For this review, take the finished solid that the model builds, in its own axes (mm). Face numbers are marked on the shaded views. Give positions to 0.01 mm unless a question says otherwise; leave off trailing zeros. Write each loop counter-clockwise with the first axis right and the second up, starting at its lowest first coordinate (ties: lowest second). Pieces come first, ordered by that corner, then holes. Notation, with made-up numbers: M -25,88 L 31,88 A17 cw 31,105 Z; hole C -14.5,-6.5 d5. An arc over 180 degrees is marked long. One line per item, written item: value. Start each with the question number.
Item 1: Consider section A-A, the plane x = 0. Write out the cut boundary in (y, z), and give its area (3 significant figures).
Item 2: Consider section B-B, the plane z = 6.5. Give the number of separate pieces and of enclosed holes in the cut face, and give its area (3 significant figures).
Item 3: Mouldability with a two-part tool opening along X and no side actions: class the marked faces 1 and 2 as released by +X, released by -X, zero draft, split by the parting line, or undercut.
Item 4: To check wall thickness, follow probe 1 along X at (y, z) = (1, 9.25); probe 2 along X at (y, z) = (-29, 6.75); probe 3 along Y at (x, z) = (-25, 4). State the ranges of each line that lie inside material, in increasing order.
Item 5: Clearance check with flat-ended pins moving along their axes: pin 1 Ø5 at (y, z) = (27.5, 5.5) entering from -X; pin 2 Ø5 at (x, y) = (25.5, -5) entering from +Z; pin 3 Ø4 at (y, z) = (-27, 7) entering from +X; pin 4 Ø3 at (x, z) = (-32, 1.5) entering from -Y. State where each tip first meets the part, or that it passes through.
```python
from build123d import *

# Parameters (mm, degrees)
SKETCH_8_R      = 5.308589755
SKETCH_8_R_2    = 9.5
EXTRUDE_1_DEPTH = 10


with BuildPart() as part:
    # 草图8 → 凸台-拉伸1 (new body)
    with BuildSketch(Plane.XY):
        with BuildLine():
            ThreePointArc((44.955555556, -1.999506112), (43, 0), (44.955555556, 1.999506112))
            ThreePointArc((44.955555556, 1.999506112), (44.861280018, 3.530659308), (44.714869736, 5.05770941))
            ThreePointArc((44.714869736, 5.05770941), (42.470598646, 6.726681997), (44.089286398, 9.007487158))
            ThreePointArc((44.089286398, 9.007487158), (43.756646418, 10.505041374), (43.373155424, 11.990387341))
            ThreePointArc((43.373155424, 11.990387341), (40.895430201, 13.287730758), (42.137392686, 15.793673975))
            ThreePointArc((42.137392686, 15.793673975), (41.574578963, 17.220754456), (40.963450077, 18.627822142))
            ThreePointArc((40.963450077, 18.627822142), (38.31328054, 19.521591489), (39.14793652, 22.190968124))
            ThreePointArc((39.14793652, 22.190968124), (38.368807396, 23.512435412), (37.54508864, 24.806578139))
            ThreePointArc((37.54508864, 24.806578139), (34.787730758, 25.274765849), (35.194528232, 28.041846989))
            ThreePointArc((35.194528232, 28.041846989), (34.218268452, 29.225162175), (33.202242516, 30.374513855))
            ThreePointArc((33.202242516, 30.374513855), (30.405591591, 30.405591591), (30.374513855, 33.202242516))
            ThreePointArc((30.374513855, 33.202242516), (29.225162175, 34.218268452), (28.041846989, 35.194528232))
            ThreePointArc((28.041846989, 35.194528232), (25.274765849, 34.787730758), (24.806578139, 37.54508864))
            ThreePointArc((24.806578139, 37.54508864), (23.512435412, 38.368807396), (22.190968124, 39.14793652))
            ThreePointArc((22.190968124, 39.14793652), (19.521591489, 38.31328054), (18.627822142, 40.963450077))
            ThreePointArc((18.627822142, 40.963450077), (17.220754456, 41.574578963), (15.793673975, 42.137392686))
            ThreePointArc((15.793673975, 42.137392686), (13.287730758, 40.895430201), (11.990387341, 43.373155424))
            ThreePointArc((11.990387341, 43.373155424), (10.505041374, 43.756646418), (9.007487158, 44.089286398))
            ThreePointArc((9.007487158, 44.089286398), (6.726681997, 42.470598646), (5.05770941, 44.714869736))
            ThreePointArc((5.05770941, 44.714869736), (3.530659308, 44.861280018), (1.999506112, 44.955555556))
            ThreePointArc((1.999506112, 44.955555556), (0, 43), (-1.999506112, 44.955555556))
            ThreePointArc((-1.999506112, 44.955555556), (-3.530659308, 44.861280018), (-5.05770941, 44.714869736))
            ThreePointArc((-5.05770941, 44.714869736), (-5.044095711, 44.580728744), (-5.039550927, 44.445975327))
            ThreePointArc((-5.039550927, 44.445975327), (-6.860487337, 42.454007398), (-9.007487158, 44.089286398))
            ThreePointArc((-9.007487158, 44.089286398), (-10.505041374, 43.756646418), (-11.990387341, 43.373155424))
            ThreePointArc((-11.990387341, 43.373155424), (-11.927033485, 43.088442863), (-11.905764747, 42.797543233))
            ThreePointArc((-11.905764747, 42.797543233), (-13.570965148, 40.825765044), (-15.793673975, 42.137392686))
            ThreePointArc((-15.793673975, 42.137392686), (-17.220754456, 41.574578963), (-18.627822142, 40.963450077))
            ThreePointArc((-18.627822142, 40.963450077), (-18.479764717, 40.540545937), (-18.429572488, 40.095293588))
            ThreePointArc((-18.429572488, 40.095293588), (-19.941101031, 38.155861807), (-22.190968124, 39.14793652))
            ThreePointArc((-22.190968124, 39.14793652), (-23.512435412, 38.368807396), (-24.806578139, 37.54508864))
            ThreePointArc((-24.806578139, 37.54508864), (-24.541473285, 37.002624685), (-24.450336353, 36.405764747))
            ThreePointArc((-24.450336353, 36.405764747), (-25.811204626, 34.510636615), (-28.041846989, 35.194528232))
            ThreePointArc((-28.041846989, 35.194528232), (-29.225162175, 34.218268452), (-30.374513855, 33.202242516))
            ThreePointArc((-30.374513855, 33.202242516), (-29.963655564, 32.564592842), (-29.819805153, 31.819805153))
            ThreePointArc((-29.819805153, 31.819805153), (-31.033953617, 29.980664767), (-33.202242516, 30.374513855))
            ThreePointArc((-33.202242516, 30.374513855), (-34.218268452, 29.225162175), (-35.194528232, 28.041846989))
            ThreePointArc((-35.194528232, 28.041846989), (-34.613772416, 27.338459928), (-34.405764747, 26.450336353))
            ThreePointArc((-34.405764747, 26.450336353), (-35.478038437, 24.678522623), (-37.54508864, 24.806578139))
            ThreePointArc((-37.54508864, 24.806578139), (-38.368807396, 23.512435412), (-39.14793652, 22.190968124))
            ThreePointArc((-39.14793652, 22.190968124), (-38.378506744, 21.455556373), (-38.095293588, 20.429572488))
            ThreePointArc((-38.095293588, 20.429572488), (-39.031412246, 18.736009236), (-40.963450077, 18.627822142))
            ThreePointArc((-40.963450077, 18.627822142), (-41.574578963, 17.220754456), (-42.137392686, 15.793673975))
            ThreePointArc((-42.137392686, 15.793673975), (-41.166546438, 15.063283409), (-40.797543233, 13.905764747))
            ThreePointArc((-40.797543233, 13.905764747), (-41.604066041, 12.300893353), (-43.373155424, 11.990387341))
            ThreePointArc((-43.373155424, 11.990387341), (-43.756646418, 10.505041374), (-44.089286398, 9.007487158))
            ThreePointArc((-44.089286398, 9.007487158), (-42.910824217, 8.321467879), (-42.445975327, 7.039550927))
            ThreePointArc((-42.445975327, 7.039550927), (-43.130260468, 5.533265957), (-44.714869736, 5.05770941))
            ThreePointArc((-44.714869736, 5.05770941), (-44.861280018, 3.530659308), (-44.955555556, 1.999506112))
            ThreePointArc((-44.955555556, 1.999506112), (-43.570159294, 1.398411798), (-43, 0))
            ThreePointArc((-43, 0), (-43.570159294, -1.398411798), (-44.955555556, -1.999506112))
            ThreePointArc((-44.955555556, -1.999506112), (-44.861280018, -3.530659308), (-44.714869736, -5.05770941))
            ThreePointArc((-44.714869736, -5.05770941), (-43.130260468, -5.533265957), (-42.445975327, -7.039550927))
            ThreePointArc((-42.445975327, -7.039550927), (-42.910824217, -8.321467879), (-44.089286398, -9.007487158))
            ThreePointArc((-44.089286398, -9.007487158), (-43.756646418, -10.505041374), (-43.373155424, -11.990387341))
            ThreePointArc((-43.373155424, -11.990387341), (-41.604066041, -12.300893353), (-40.797543233, -13.905764747))
            ThreePointArc((-40.797543233, -13.905764747), (-41.166546438, -15.063283409), (-42.137392686, -15.793673975))
            ThreePointArc((-42.137392686, -15.793673975), (-41.574578963, -17.220754456), (-40.963450077, -18.627822142))
            ThreePointArc((-40.963450077, -18.627822142), (-39.031412246, -18.736009236), (-38.095293588, -20.429572488))
            ThreePointArc((-38.095293588, -20.429572488), (-38.378506744, -21.455556373), (-39.14793652, -22.190968124))
            ThreePointArc((-39.14793652, -22.190968124), (-38.368807396, -23.512435412), (-37.54508864, -24.806578139))
            ThreePointArc((-37.54508864, -24.806578139), (-35.478038437, -24.678522623), (-34.405764747, -26.450336353))
            ThreePointArc((-34.405764747, -26.450336353), (-34.613772416, -27.338459928), (-35.194528232, -28.041846989))
            ThreePointArc((-35.194528232, -28.041846989), (-34.218268452, -29.225162175), (-33.202242516, -30.374513855))
            ThreePointArc((-33.202242516, -30.374513855), (-31.033953617, -29.980664767), (-29.819805153, -31.819805153))
            ThreePointArc((-29.819805153, -31.819805153), (-29.963655564, -32.564592842), (-30.374513855, -33.202242516))
            ThreePointArc((-30.374513855, -33.202242516), (-29.225162175, -34.218268452), (-28.041846989, -35.194528232))
            ThreePointArc((-28.041846989, -35.194528232), (-25.811204626, -34.510636615), (-24.450336353, -36.405764747))
            ThreePointArc((-24.450336353, -36.405764747), (-24.541473285, -37.002624685), (-24.806578139, -37.54508864))
            ThreePointArc((-24.806578139, -37.54508864), (-23.512435412, -38.368807396), (-22.190968124, -39.14793652))
            ThreePointArc((-22.190968124, -39.14793652), (-19.941101031, -38.155861807), (-18.429572488, -40.095293588))
            ThreePointArc((-18.429572488, -40.095293588), (-18.479764717, -40.540545937), (-18.627822142, -40.963450077))
            ThreePointArc((-18.627822142, -40.963450077), (-17.220754456, -41.574578963), (-15.793673975, -42.137392686))
            ThreePointArc((-15.793673975, -42.137392686), (-13.570965148, -40.825765044), (-11.905764747, -42.797543233))
            ThreePointArc((-11.905764747, -42.797543233), (-11.927033485, -43.088442863), (-11.990387341, -43.373155424))
            ThreePointArc((-11.990387341, -43.373155424), (-10.505041374, -43.756646418), (-9.007487158, -44.089286398))
            ThreePointArc((-9.007487158, -44.089286398), (-6.860487337, -42.454007398), (-5.039550927, -44.445975327))
            ThreePointArc((-5.039550927, -44.445975327), (-5.044095711, -44.580728744), (-5.05770941, -44.714869736))
            ThreePointArc((-5.05770941, -44.714869736), (-3.530659308, -44.861280018), (-1.999506112, -44.955555556))
            ThreePointArc((-1.999506112, -44.955555556), (0, -43), (1.999506112, -44.955555556))
            ThreePointArc((1.999506112, -44.955555556), (3.530659308, -44.861280018), (5.05770941, -44.714869736))
            ThreePointArc((5.05770941, -44.714869736), (6.726681997, -42.470598646), (9.007487158, -44.089286398))
            ThreePointArc((9.007487158, -44.089286398), (10.505041374, -43.756646418), (11.990387341, -43.373155424))
            ThreePointArc((11.990387341, -43.373155424), (13.287730758, -40.895430201), (15.793673975, -42.137392686))
            ThreePointArc((15.793673975, -42.137392686), (17.220754456, -41.574578963), (18.627822142, -40.963450077))
            ThreePointArc((18.627822142, -40.963450077), (19.521591489, -38.31328054), (22.190968124, -39.14793652))
            ThreePointArc((22.190968124, -39.14793652), (23.512435412, -38.368807396), (24.806578139, -37.54508864))
            ThreePointArc((24.806578139, -37.54508864), (25.274765849, -34.787730758), (28.041846989, -35.194528232))
            ThreePointArc((28.041846989, -35.194528232), (29.225162175, -34.218268452), (30.374513855, -33.202242516))
            ThreePointArc((30.374513855, -33.202242516), (30.405591591, -30.405591591), (33.202242516, -30.374513855))
            ThreePointArc((33.202242516, -30.374513855), (34.218268452, -29.225162175), (35.194528232, -28.041846989))
            ThreePointArc((35.194528232, -28.041846989), (34.787730758, -25.274765849), (37.54508864, -24.806578139))
            ThreePointArc((37.54508864, -24.806578139), (38.368807396, -23.512435412), (39.14793652, -22.190968124))
            ThreePointArc((39.14793652, -22.190968124), (38.31328054, -19.521591489), (40.963450077, -18.627822142))
            ThreePointArc((40.963450077, -18.627822142), (41.574578963, -17.220754456), (42.137392686, -15.793673975))
            ThreePointArc((42.137392686, -15.793673975), (40.895430201, -13.287730758), (43.373155424, -11.990387341))
            ThreePointArc((43.373155424, -11.990387341), (43.756646418, -10.505041374), (44.089286398, -9.007487158))
            ThreePointArc((44.089286398, -9.007487158), (42.470598646, -6.726681997), (44.714869736, -5.05770941))
            ThreePointArc((44.714869736, -5.05770941), (44.861280018, -3.530659308), (44.955555556, -1.999506112))
        make_face()
        with Locations((0, -26.450336353)):
            Circle(SKETCH_8_R, mode=Mode.SUBTRACT)
        with Locations((-26.450336353, 0)):
            Circle(SKETCH_8_R, mode=Mode.SUBTRACT)
        Circle(SKETCH_8_R_2, mode=Mode.SUBTRACT)
        with Locations((0, 26.450336353)):
            Circle(SKETCH_8_R, mode=Mode.SUBTRACT)
        with Locations((26.450336353, 0)):
            Circle(SKETCH_8_R, mode=Mode.SUBTRACT)
    extrude(amount=EXTRUDE_1_DEPTH)


solid = part.part
```
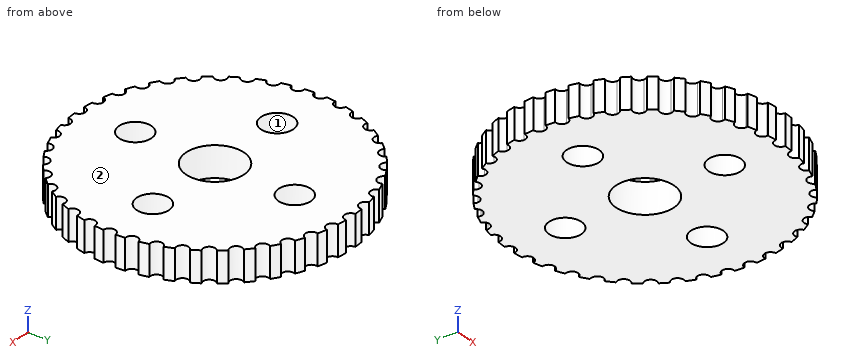
Model answer:
1. outline: M -43,0 L -31.76,0 L -31.76,10 L -43,10 Z; M -21.14,0 L -9.5,0 L -9.5,10 L -21.14,10 Z; M 9.5,0 L 21.14,0 L 21.14,10 L 9.5,10 Z; M 31.76,0 L 43,0 L 43,10 L 31.76,10 Z
1. area: 458 mm2
2. separate pieces: 1
2. enclosed holes: 5
2. area: 5,480 mm2
3. face 1: undercut
3. face 2: zero draft
4. probe 1: x = -43.27 to -31.66, -21.24 to -9.45, 9.45 to 21.24, 31.66 to 43.27
4. probe 2: x = -34.41 to -4.66, 4.66 to 34.41
4. probe 3: y = -35.03 to -5.11, 5.11 to 35.03
5. pin 1: stops at x = -35.19
5. pin 2: stops at z = 10
5. pin 3: stops at x = 35.19
5. pin 4: stops at y = -30.37
